Geometry check sheet. Reference: drawing and pictorial views, mm from the part's lowest x, y, z. A direction names the side the tool comes from. Coordinates: 2 decimals unless noted, no trailing zeros. Write each loop counter-clockwise with the first axis right and the second up, starting at its lowest first coordinate (ties: lowest second). Pieces come first, ordered by that corner, then holes. Notation, with made-up numbers: (-2.75, -23.75) -> (9.25, -23.75) arc R30 cw to (9.25, 10.25) -> close; hole circle Ø7 at (-30, 63). An arc over 180 degrees is marked (long way). Answer in a Markdown table with one row per item.
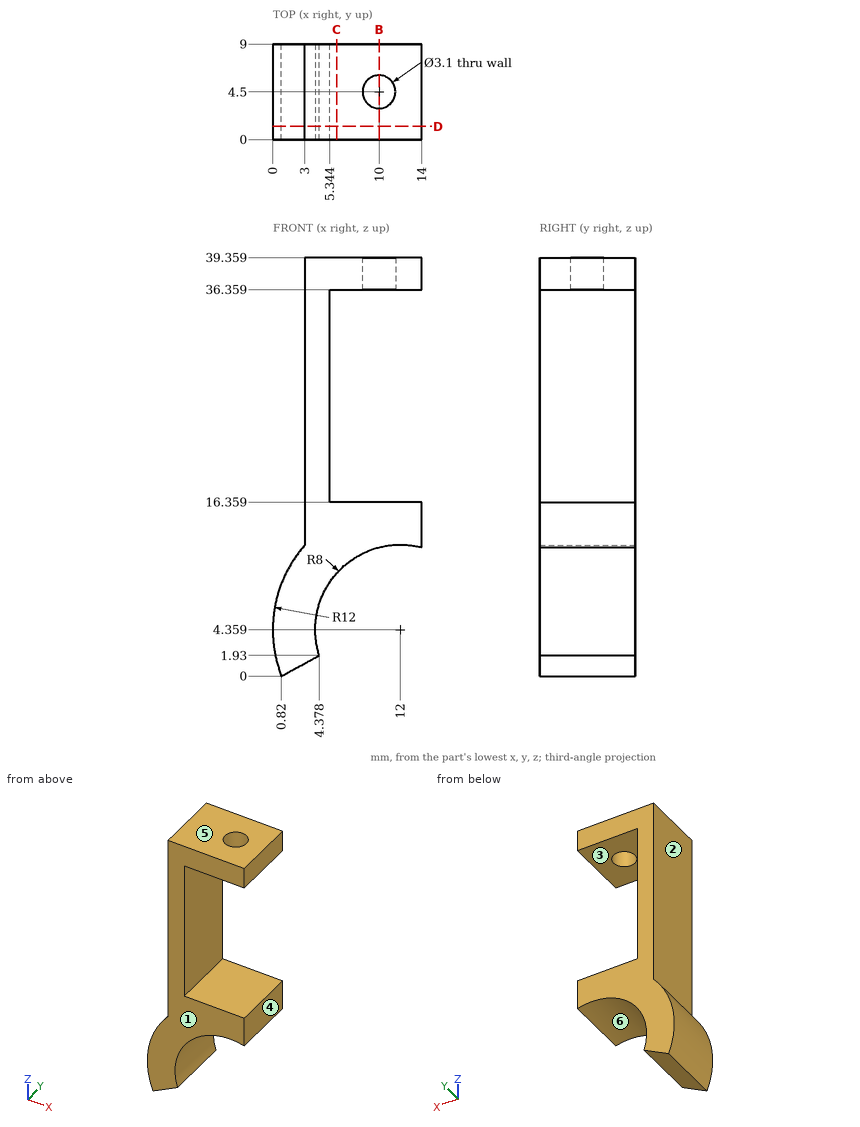
1. Thickness scan on line 1 (Y direction, x = 10, z = 38.15); line 2 (Z direction, x = 11.75, y = 5.25) (1 decimal); line 3 (X direction, y = 5, z = 15). Record the ranges inside material, lowest first. Write a range as from..to.
Geometry says:
| item | result |
|---|---|
| line 1 | 0..2.95, 6.05..9 |
| line 2 | 12.4..16.4, 36.4..39.4 |
| line 3 | 3..14 |
2. Depth check by flat-ended pin: P1, Ø4.5, axis at y = 3, z = 21.5, coming from the +X side; P2, Ø3, axis at x = 10, y = 4.5, coming from the -Z side; P3, Ø8, axis at x = 12, z = 4.5, coming from the +Y side. Enter the tip coordinate at first touch or a pass-through.
Geometry says:
| item | result |
|---|---|
| P1 | x = 5.34 |
| P2 | z = 11.55 |
| P3 | through |
3. Mould release check, pull along Z, two halves, no side actions. Record for the marked faces 4, 5 and 6: released by +Z, released by -Z, zero draft, split by the parting line, or undercut.
Geometry says:
| item | result |
|---|---|
| face 4 | zero draft |
| face 5 | released by +Z |
| face 6 | undercut |
4. Section check C-C, the plane x = 6. Record the boundary of the cut face in (y, z).
Geometry says:
| item | result |
|---|---|
| outline | (0, 9.65) -> (9, 9.65) -> (9, 16.36) -> (0, 16.36) -> close; (0, 36.36) -> (9, 36.36) -> (9, 39.36) -> (0, 39.36) -> close |
5. Section check D-D, the plane y = 1.25. Record the boundary of the cut face in (x, z) (1 decimal), plus the area to 3 significant figures.
Geometry says:
| item | result |
|---|---|
| outline | (0.8, 0) -> (4.4, 1.9) arc R8 cw to (14, 12.1) -> (14, 16.4) -> (5.3, 16.4) -> (5.3, 36.4) -> (14, 36.4) -> (14, 39.4) -> (3, 39.4) -> (3, 12.3) arc R12 ccw to start |
| area | 176 mm^2 |
6. Tool access check on the marked faces 1, 2 and 3. Record the directions out of +Z, -Z, +X, -X, +Y, -Y that give a thin tool (end or side, any length) a straight path to the whole face; none if there is none.
Geometry says:
| item | result |
|---|---|
| face 1 | +Z, -Z, +X, -X, -Y |
| face 2 | +Z, -X, +Y, -Y |
| face 3 | +X, +Y, -Y |
7. Section check B-B, the plane x = 10. State how many separate pieces and enclosed holes the cut face has.
Geometry says:
| item | result |
|---|---|
| separate pieces | 3 |
| enclosed holes | 0 |
